Print and shaded views of the part. All mm, measured from the part's lowest x, y and z. A direction names the side the tool comes from. Round coordinates to 2 decimals unless told otherwise and drop trailing zeros. Loops run counter-clockwise (first coordinate to the right, second up) from the corner with the lowest first, then second, coordinate; pieces in that order, holes last. Notation, with made-up numbers: (25, 58) - (33, 58) arc R17 ccw to (33, 80) - close; hole circle Ø5 at (32, 40). An arc over 180 degrees is marked (long way). Use one line per item in the form item = value.
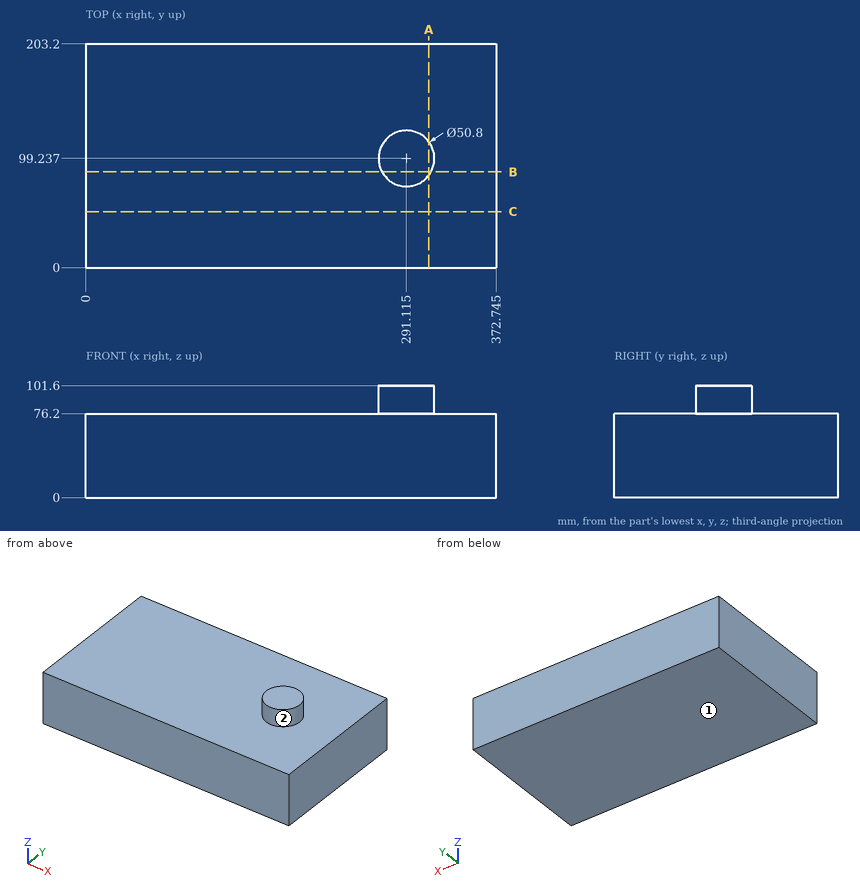
1) Slice it at A-A (x = 311.5). Write the cut outline in (y, z).
Report:
outline = (0, 0) - (203.2, 0) - (203.2, 76.2) - (114.39, 76.2) - (114.39, 101.6) - (84.08, 101.6) - (84.08, 76.2) - (0, 76.2) - close
2) Tool access for the marked faces 1 and 2: list every direction of +Z, -Z, +X, -X, +Y, -Y with a clear straight run to the whole face (end or side of a thin tool).
Report:
face_1 = -Z, +X, -X, +Y, -Y
face_2 = +Z
3) Slice it at C-C (y = 51). Write the cut outline in (x, z) (1 decimal), plus the area to 3 significant figures.
Report:
outline = (0, 0) - (372.7, 0) - (372.7, 76.2) - (0, 76.2) - close
area = 28,400 mm^2
4) Drill centre lines: probe 1 along Z at (x, y) = (89, 132.5); probe 2 along X at (y, z) = (120, 84) (1 decimal). Where is each one in solid material? Low to high.
Report:
probe_1 = 0 to 76.2
probe_2 = 276.5 to 305.7
5) Slice it at B-B (y = 87). Write the cut outline in (x, z) (1 decimal).
Report:
outline = (0, 0) - (372.7, 0) - (372.7, 76.2) - (313.4, 76.2) - (313.4, 101.6) - (268.9, 101.6) - (268.9, 76.2) - (0, 76.2) - close
